Here's how the part is built. I have some questions about the finished solid (model axes, mm). A direction names the side the tool comes from. Round coordinates to 2 decimals unless told otherwise and drop trailing zeros. Write each loop counter-clockwise with the first axis right and the second up, starting at its lowest first coordinate (ties: lowest second). Pieces come first, ordered by that corner, then holes. Notation, with made-up numbers: M 68.5,57.25 L 118.5,57.25 A19 ccw 118.5,61.25 Z; hole C 79,56 d1. An arc over 180 degrees is marked long. Write item = value, one per line. Start each with the question number.
(1) Will these pins go through, and if not, where does the flat tip stop? pin 1 Ø1.5 at (x, y) = (130, -317) entering from -Z; pin 2 Ø4 at (x, z) = (165.63, 40.4) entering from +Y; pin 3 Ø1.5 at (x, y) = (162.5, -269.5) entering from +Z.
(2) On a 3-axis mill with a long thin cutter (end or side, diameter ignored), from which of +Z, -Z, +X, -X, +Y, -Y can I reach the whole of each face in a straight line? I mean faces 4 (the cylindrical face through (133.97, -78.59, 21.26)), 5 (the flat face through (145, -63.378, 41)). Say none if no direction works.
(3) If we mould it in two halves opening along Z, with no side actions, what happens to faces 1 (the cylindrical face through (153.194, -78.588, 22.754)), 2 (the flat face through (145, -363.378, 41)), 3 (the cylindrical face through (115.66, -211.28, 39.08))? For each: released by +Z, released by -Z, zero draft, split by the parting line, or undercut.
(4) I want a section at A-A (y = -113). List the corners of the cut face in (x, z) for me (3 decimals).
(5) I want a section at B-B (z = 15.5). List the corners of the cut face in (x, y) for me.
(6) I want a section at C-C (z = 49). List the corners of the cut face in (x, y) for me.
(7) I need wall thicknesses on line 1 along Z through (x, y) = (147.5, -172); line 2 along Z through (x, y) = (122.5, -280); line 3 along X through (y, z) = (-332, 41.5). Which ranges of each line are inside material? Lowest first, please.
Autodesk Inventor part; units mm, degrees
ref_plane "YZ Plane" through (0, 0, 0) normal (1, 0, 0) x (0, 1, 0)
ref_plane "XZ Plane" through (0, 0, 0) normal (0, 1, 0) x (-1, 0, 0)
ref_plane "XY Plane" through (0, 0, 0) normal (0, 0, 1) x (1, 0, 0)
ref_plane "Work Plane1" through (145.6317, -63.3782, 40.395) normal (0, -1, 0) x (1, 0, 0)
sketch "Sketch1" plane through (145.6317, -63.3782, 40.395) normal (0, -1, 0) x (1, 0, 0)
  circle A0 centre (0, 0) radius 60
  circle A1 centre (0, 0) radius 30
  point P0 (-145.6317, -40.395)
  dimension "d0" = 60
extrude "Extrusion1" add sketch "Sketch1" along normal blind 300 contours A1
sketch "Sketch2" plane through (145.6317, -63.3782, 40.395) normal (0, 1, 0) x (1, 0, 0)
  circle A0 centre (-20, 0) radius 3.3
  circle A1 centre (-10, 17.3205) radius 3.3
  circle A2 centre (10, 17.3205) radius 5.5
  circle A3 centre (10, 17.3205) radius 3.3
  circle A4 centre (20, 0) radius 3.3
  circle A5 centre (10, -17.3205) radius 3.3
  circle A6 centre (-10, -17.3205) radius 3.3
  point P0 (-145.6317, 40.395)
hole "Hole1" at (135.6317, -63.3782, 23.0745) at (155.6317, -63.3782, 23.0745) at (165.6317, -63.3782, 40.395) at (155.6317, -63.3782, 57.7155) at (135.6317, -63.3782, 57.7155) at (125.6317, -63.3782, 40.395) direction (0, -1, 0) diameter 4.917 depth 30 tip angle 118
sketch "Sketch3" plane through (145.6317, -63.3782, 40.395) normal (0, 1, 0) x (1, 0, 0)
  point P0 (-145.6317, 40.395)
  point P1 (0, 0)
properties part number "base_stange" material "Copper"
Returned:
q1.pin_1 = 14.35
q1.pin_2 = -93.65
q1.pin_3 = 65.7
q2.face_4 = +Y
q2.face_5 = +Z, -Z, +X, -X, +Y
q3.face_1 = undercut
q3.face_2 = zero draft
q3.face_3 = split by the parting line
q4.outline = C 145.632,40.395 d60
q5.outline = M 128.89,-363.38 L 162.37,-363.38 L 162.37,-63.38 L 128.89,-63.38 Z
q6.outline = M 116.89,-363.38 L 174.37,-363.38 L 174.37,-63.38 L 116.89,-63.38 Z
q7.line_1 = 10.45 to 70.34
q7.line_2 = 21.29 to 59.5
q7.line_3 = 115.65 to 175.61
